Can you work these out from the model? Positions are in its coordinate system, mm. Round coordinates to 2 decimals unless told otherwise and drop trailing zeros. Write each loop counter-clockwise with the first axis right and the second up, starting at its lowest first coordinate (ties: lowest second). Pieces come first, ordered by that corner, then holes. Notation, with made-up numbers: M 58,-37.75 L 114,-37.75 A32 ccw 114,-9.75 Z; hole C -4,77.5 d7. An arc over 180 degrees is marked long. Answer as a JSON object with one key per item and string values. Group by question number.
1) Suppose I cut it at B-B, the plane x = -8. Write out the boundary of the cut face in (y, z).
2) If we mould it in two halves opening along X, with no side actions, what happens to faces 1 (the cylindrical face through (0.298, 33.396, 2.465)), 2 (the flat face through (7, 3, 5)), 3 (the cylindrical face through (19.39, -27.19, 2.46))? For each: +X half, -X half, draft (parallel to the pull), parting line (faces both ways), or undercut.
3) Please list where these lines run through material, in increasing order: L1, parallel to Y at x = -20.5, z = 3.55; L2, parallel to X at y = 16.5, z = 3.65; L3, parallel to Y at x = -15.5, z = 3.2. Write a range as [from, to].
4) Suppose I cut it at A-A, the plane x = 23. Write out the boundary of the cut face in (y, z), and give its area (3 significant figures).
5) Suppose I cut it at D-D, the plane z = 3.1. Write out the boundary of the cut face in (x, y) (3 decimals), and give its area (3 significant figures).
6) I'm going to push flat-ended pins straight in: pin 1 Ø1.5 at (y, z) = (9.5, 3.5) entering from +X; pin 2 Ø1 at (y, z) = (-15.5, 0.5) entering from +X; pin 3 Ø1.5 at (x, z) = (10, 3) entering from +Y; pin 4 Ø1.8 at (x, y) = (-4.1, 7.1) entering from -Z. Where does each tip first touch, or does it pass through?
7) Suppose I cut it at C-C, the plane y = 0. Write out the boundary of the cut face in (x, z), and give its area (3 significant figures).
from build123d import *

# Parameters (mm, degrees)
ESTRUSIONE_ESTRUSIONE1_DEPTH = 5
SCHIZZO2_R                   = 1
TAGLIO_ESTRUSIONE1_DEPTH     = 5
SCHIZZO1_4_R                 = 5
ESTRUSIONE_ESTRUSIONE2_DEPTH = 5
SCHIZZO1_5_R                 = 5
TAGLIO_ESTRUSIONE2_DEPTH     = 5


with BuildPart() as part:
    # Schizzo1 → Estrusione-Estrusione1 (new body)
    with BuildSketch(Plane.XY):
        with BuildLine():
            Line((-10.272621339, 18.466394679), (-6.769041701, 9.316786616))
            Line((-6.769041701, 9.316786616), (-14.388170422, 15.476273245))
            ThreePointArc((-14.388170422, 15.476273245), (-31.765287644, 10.321167612), (-20.736999563, -4.063413683))
            Line((-20.736999563, -4.063413683), (-10.952539543, -3.558695821))
            Line((-10.952539543, -3.558695821), (-19.164999696, -8.901531795))
            ThreePointArc((-19.164999696, -8.901531795), (-19.632027427, -27.021167612), (-2.543549215, -20.977722446))
            Line((-2.543549215, -20.977722446), (0, -11.516181589))
            Line((0, -11.516181589), (2.543549215, -20.977722446))
            ThreePointArc((2.543549215, -20.977722446), (19.632027427, -27.021167612), (19.164999696, -8.901531795))
            Line((19.164999696, -8.901531795), (10.952539543, -3.558695821))
            Line((10.952539543, -3.558695821), (20.736999563, -4.063413683))
            ThreePointArc((20.736999563, -4.063413683), (31.765287644, 10.321167612), (14.388170422, 15.476273245))
            Line((14.388170422, 15.476273245), (6.769041701, 9.316786616))
            Line((6.769041701, 9.316786616), (10.272621339, 18.466394679))
            ThreePointArc((10.272621339, 18.466394679), (0, 33.4), (-10.272621339, 18.466394679))
        make_face()
    extrude(amount=ESTRUSIONE_ESTRUSIONE1_DEPTH)

    # Schizzo2 → Taglio-Estrusione1 (cut)
    with BuildSketch(Plane.XY.offset(5)):
        with Locations((8.2, 0)):
            Circle(SCHIZZO2_R)
        with Locations((4.1, -7.101408311)):
            Circle(SCHIZZO2_R)
        with Locations((-4.1, -7.101408311)):
            Circle(SCHIZZO2_R)
        with Locations((-8.2, 0)):
            Circle(SCHIZZO2_R)
        with Locations((-4.1, 7.101408311)):
            Circle(SCHIZZO2_R)
        with Locations((4.1, 7.101408311)):
            Circle(SCHIZZO2_R)
    extrude(amount=-TAGLIO_ESTRUSIONE1_DEPTH, mode=Mode.SUBTRACT)

    # Schizzo1<4> → Estrusione-Estrusione2 (add)
    with BuildSketch(Plane.XY):
        Circle(SCHIZZO1_4_R)
    extrude(amount=ESTRUSIONE_ESTRUSIONE2_DEPTH)

    # Schizzo1<5> → Taglio-Estrusione2 (cut)
    with BuildSketch(Plane.XY):
        Circle(SCHIZZO1_5_R)
    extrude(amount=TAGLIO_ESTRUSIONE2_DEPTH, mode=Mode.SUBTRACT)


solid = part.part
Results:
{
 "1": {"outline": "M -27.83,0 L -0.98,0 L -0.98,5 L -27.83,5 Z; M 0.98,0 L 10.31,0 L 10.31,5 L 0.98,5 Z; M 12.53,0 L 29.95,0 L 29.95,5 L 12.53,5 Z"},
 "2": {"face 1": "parting line", "face 2": "draft", "face 3": "undercut"},
 "3": {"L1": "[-26.32, -9.92], [-4.05, 17.89]", "L2": "[-26.71, -15.89], [-9.52, 9.52], [15.89, 26.71]", "L3": "[-28.87, -6.52], [-3.79, 16.27]"},
 "4": {"outline": "M -23.05,0 L -13.19,0 L -13.19,5 L -23.05,5 Z; M -3.95,0 L 17.79,0 L 17.79,5 L -3.95,5 Z", "area": "158 mm^2"},
 "5": {"outline": "M -20.737,-4.063 L -10.953,-3.559 L -19.165,-8.902 A11 ccw long -2.544,-20.978 L 0,-11.516 L 2.544,-20.978 A11 ccw long 19.165,-8.902 L 10.953,-3.559 L 20.737,-4.063 A11 ccw long 14.388,15.476 L 6.769,9.317 L 10.273,18.466 A11 ccw long -10.273,18.466 L -6.769,9.317 L -14.388,15.476 A11 ccw long Z; hole C -8.2,0 d2; hole C -4.1,-7.101 d2; hole C -4.1,7.101 d2; hole C 0,0 d10; hole C 4.1,-7.101 d2; hole C 4.1,7.101 d2; hole C 8.2,0 d2", "area": "2,370 mm^2"},
 "6": {"pin 1": "x = 32.15", "pin 2": "x = 23.96", "pin 3": "y = 28.35", "pin 4": "through"},
 "7": {"outline": "M -29.85,0 L -9.2,0 L -9.2,5 L -29.85,5 Z; M -7.2,0 L -5,0 L -5,5 L -7.2,5 Z; M 5,0 L 7.2,0 L 7.2,5 L 5,5 Z; M 9.2,0 L 29.85,0 L 29.85,5 L 9.2,5 Z", "area": "229 mm^2"}
}
